Can you work these out from the model? Positions are in its coordinate system, mm. Face numbers are marked on the shaded views. Give positions to 0.01 mm unless a question says otherwise; leave off trailing zeros. Write each loop counter-clockwise with the first axis right and the second up, starting at its lowest first coordinate (ties: lowest second). Pieces come first, ordered by that corner, then holes. Notation, with made-up numbers: (12, 81) -> (65, 81) arc R29 cw to (65, 103) -> close; hole circle Ø4 at (54, 84). An arc over 180 degrees is marked (long way). One line per item, written item: value.
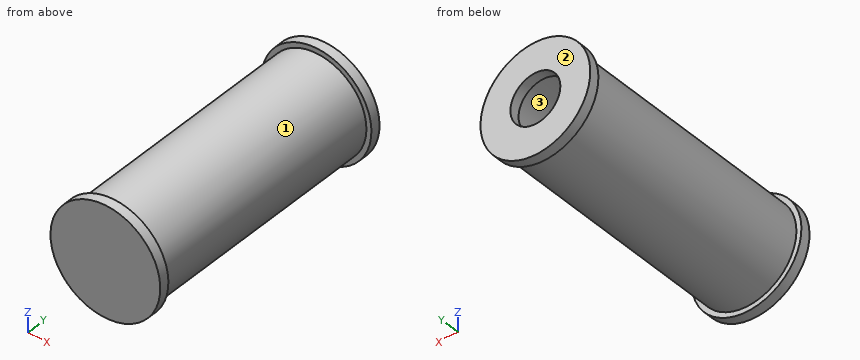
from build123d import *

# Parameters (mm, degrees)
SKETCH1_W           = 2
SKETCH1_H           = 100
SKETCH2_R           = 22
BOSS_EXTRUDE1_DEPTH = 4
BOSS_EXTRUDE2_START = 4
SKETCH3_R           = 22
BOSS_EXTRUDE2_DEPTH = 4
SKETCH4_R           = 10
CUT_EXTRUDE1_DEPTH  = 4


with BuildPart() as part:
    # Sketch1 → Revolve1 (revolve)
    with BuildSketch(Plane.XY, mode=Mode.PRIVATE) as revolve1_sk:
        with Locations((19, 50)):
            Rectangle(SKETCH1_W, SKETCH1_H)
    revolve(revolve1_sk.sketch.rotate(Axis((0, 0, 0), (0, 1, 0)), 90), axis=Axis((0, 0, 0), (0, 1, 0)))

    # Sketch2 → Boss-Extrude1 (add)
    with BuildSketch(Plane(origin=(0, 100, 0), x_dir=(1, 0, 0), z_dir=(0, 1, 0))):
        with Locations(Location((0, 0, 0), (0, 0, 270))):
            Circle(SKETCH2_R)
    extrude(amount=BOSS_EXTRUDE1_DEPTH)

    # Sketch3 → Boss-Extrude2 (add)
    with BuildSketch(Plane.XZ.offset(BOSS_EXTRUDE2_START)):
        with Locations(Location((0, 0, 0), (0, 0, 90))):
            Circle(SKETCH3_R)
    extrude(amount=-BOSS_EXTRUDE2_DEPTH)

    # Sketch4 → Cut-Extrude1 (cut)
    with BuildSketch(Plane(origin=(0, 104, 0), x_dir=(1, 0, 0), z_dir=(0, 1, 0))):
        with Locations(Location((0, 0, 0), (0, 0, 270))):
            Circle(SKETCH4_R)
    extrude(amount=-CUT_EXTRUDE1_DEPTH, mode=Mode.SUBTRACT)


solid = part.part
1) We'd pull the mould along X, two halves only. Please class the marked faces 1, 2 and 3: released by +X, released by -X, zero draft, split by the parting line, or undercut.
Answer list:
face 1: split by the parting line
face 2: zero draft
face 3: undercut
2) If we section it at B-B (z = 0): Write out the boundary of the cut face in (x, y), and give its area (3 significant figures).
Answer list:
outline: (-22, -4) -> (22, -4) -> (22, 0) -> (20, 0) -> (20, 100) -> (22, 100) -> (22, 104) -> (10, 104) -> (10, 100) -> (18, 100) -> (18, 0) -> (-18, 0) -> (-18, 100) -> (-10, 100) -> (-10, 104) -> (-22, 104) -> (-22, 100) -> (-20, 100) -> (-20, 0) -> (-22, 0) -> close
area: 672 mm^2
3) Will these pins go through, and if not, where does the flat tip stop? pin 1 (5 mm diameter, centred on x = -0.5, y = 24, fed in from +Z); pin 2 (3 mm diameter, centred on x = -11.5, y = 60, fed in from +Z); pin 3 (10 mm diameter, centred on y = 58.5, z = 6.5, fed in from -X).
Answer list:
pin 1: stops at z = 20
pin 2: stops at z = 17.32
pin 3: stops at x = -19.94
4) If we section it at A-A (x = 0): Write out the boundary of the cut face in (y, z).
Answer list:
outline: (-4, -22) -> (0, -22) -> (0, -20) -> (100, -20) -> (100, -22) -> (104, -22) -> (104, -10) -> (100, -10) -> (100, -18) -> (0, -18) -> (0, 18) -> (100, 18) -> (100, 10) -> (104, 10) -> (104, 22) -> (100, 22) -> (100, 20) -> (0, 20) -> (0, 22) -> (-4, 22) -> close
5) If we section it at C-C (y = 38): Write out the boundary of the cut face in (x, z), and give its area (3 significant figures).
Answer list:
outline: circle Ø40 at (0, 0); hole circle Ø36 at (0, 0)
area: 239 mm^2
6) I need wall thicknesses on L1, parallel to X at y = 69, z = 0; L2, parallel to Y at x = 13.5, z = 4; L3, parallel to X at y = 100.8, z = 0. Which ranges of each line are inside material? Lowest first, please.
Answer list:
L1: x = -20 to -18, 18 to 20
L2: y = -4 to 0, 100 to 104
L3: x = -22 to -10, 10 to 22
7) If we section it at D-D (x = -16): Write out the boundary of the cut face in (y, z), and give its area (3 significant figures).
Answer list:
outline: (-4, -15.1) -> (0, -15.1) -> (0, -12) -> (100, -12) -> (100, -15.1) -> (104, -15.1) -> (104, 15.1) -> (100, 15.1) -> (100, 12) -> (0, 12) -> (0, 15.1) -> (-4, 15.1) -> close; hole (0, -8.25) -> (100, -8.25) -> (100, 8.25) -> (0, 8.25) -> close
area: 992 mm^2
